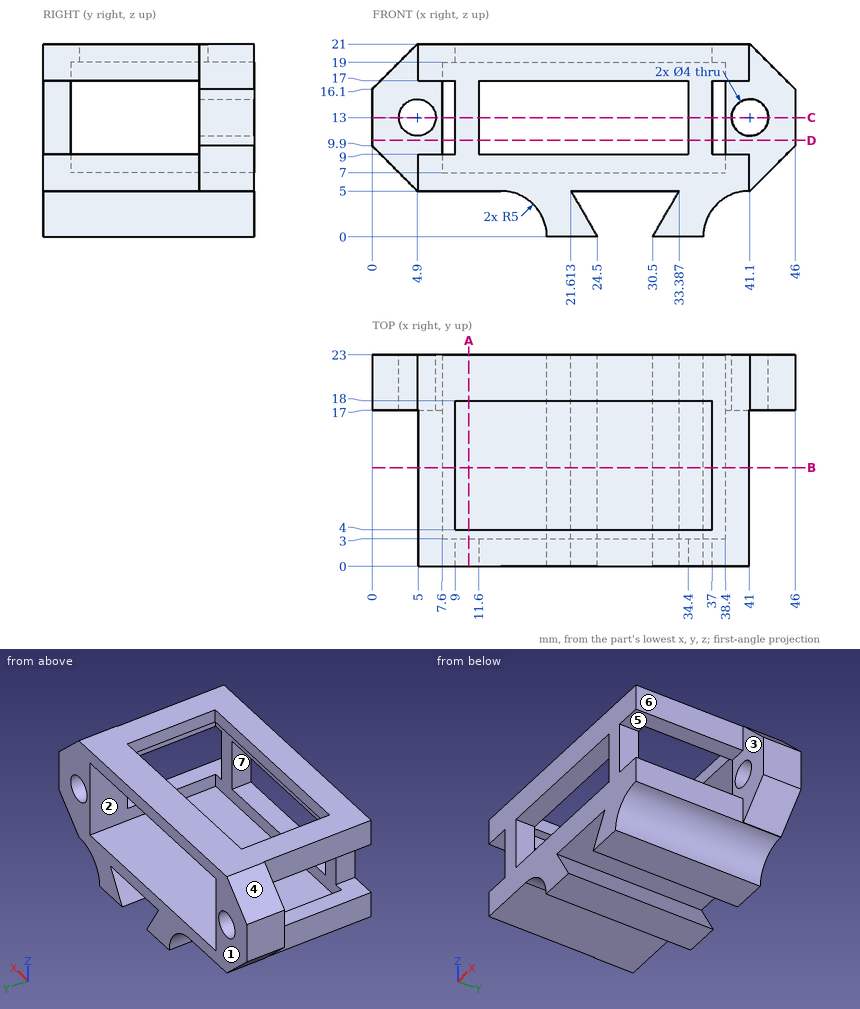
Source: three-view drawing plus pictorial views. Frame: mm from the lowest corner of the part. A direction names the side the tool comes from. Round coordinates to 2 decimals unless told otherwise and drop trailing zeros. Loops run counter-clockwise (first coordinate to the right, second up) from the corner with the lowest first, then second, coordinate; pieces in that order, holes last.
1. Contact query for flat-ended pins moving along their axis: pin 1 (3 mm diameter, centred on y = 9, z = 6, fed in from +X); pin 2 (2 mm diameter, centred on x = 6.5, y = 10.5, fed in from -Z); pin 3 (1 mm diameter, centred on y = 14, z = 20.5, fed in from -X). Output: stop coordinate, or through.
2. Section query A-A on x = 10.5. Output: boundary loops of the cut face in (y, z), and give its area (3 significant figures).
3. Section query B-B on y = 10.75. Output: boundary loops of the cut face in (x, z), and give its area (3 significant figures).
4. Access query for the marked faces 5, 6 and 7. Directions: +Z, -Z, +X, -X, +Y, -Y. A direction counts if a zero-diameter tool reaches every point of the face in a straight line with its end or side. Return the directions, or none.
5. Mould query, pull axis Z, two halves, no side actions, for the marked faces 1, 2, 3 and 4. Classes: released by +Z, released by -Z, zero draft, split by the parting line, or undercut.
6. Section query C-C on z = 13. Output: boundary loops of the cut face in (x, y).
7. Ray query, L1, parallel to X at y = 18.35, z = 13; L2, parallel to Z at x = 29.5, y = 19.25; L3, parallel to Z at x = 40, y = 16.5. Return the intervals inside material, ascending.
8. Section query D-D on z = 10.5. Output: boundary loops of the cut face in (x, y).
Answers below:
1. pin 1: stops at x = 41
1. pin 2: stops at z = 5
1. pin 3: stops at x = 5
2. outline: (0, 5) - (23, 5) - (23, 7) - (3, 7) - (3, 19) - (4, 19) - (4, 21) - (0, 21) - close; (18, 19) - (23, 19) - (23, 21) - (18, 21) - close
2. area: 100 mm2
3. outline: (5, 5) - (14, 5) arc R5 cw to (19, 0) - (24.5, 0) - (21.61, 5) - (33.39, 5) - (30.5, 0) - (36, 0) arc R5 cw to (41, 5) - (41, 9) - (38.4, 9) - (38.4, 7) - (7.6, 7) - (7.6, 9) - (5, 9) - close; (5, 17) - (7.6, 17) - (7.6, 19) - (9, 19) - (9, 21) - (5, 21) - close; (37, 19) - (38.4, 19) - (38.4, 17) - (41, 17) - (41, 21) - (37, 21) - close
3. area: 160 mm2
4. face 5: +X, -Y
4. face 6: +Z, -Z, +X, -Y
4. face 7: +Y, -Y
5. face 1: zero draft
5. face 2: undercut
5. face 3: undercut
5. face 4: released by +Z
6. outline: (0, 17) - (2.9, 17) - (2.9, 23) - (0, 23) - close; (6.9, 17) - (7.6, 17) - (7.6, 23) - (6.9, 23) - close; (9, 0) - (11.6, 0) - (11.6, 3) - (9, 3) - close; (34.4, 0) - (37, 0) - (37, 3) - (34.4, 3) - close; (38.4, 17) - (39.1, 17) - (39.1, 23) - (38.4, 23) - close; (43.1, 17) - (46, 17) - (46, 23) - (43.1, 23) - close
7. L1: x = 0 to 2.9, 6.9 to 7.6, 38.4 to 39.1, 43.1 to 46
7. L2: z = 5 to 7, 19 to 21
7. L3: z = 4.9 to 9, 17 to 21
8. outline: (0, 17) - (7.6, 17) - (7.6, 23) - (0, 23) - close; (9, 0) - (11.6, 0) - (11.6, 3) - (9, 3) - close; (34.4, 0) - (37, 0) - (37, 3) - (34.4, 3) - close; (38.4, 17) - (46, 17) - (46, 23) - (38.4, 23) - close
